Check sheet for the modelled part. Datum: model origin and axes. Units: mm. A direction names the side the tool comes from. Give positions to 0.01 mm unless a question says otherwise; leave off trailing zeros. Write each loop counter-clockwise with the first axis right and the second up, starting at its lowest first coordinate (ties: lowest second). Pieces come first, ordered by that corner, then holes. Notation, with made-up numbers: (72, 24) -> (76, 24) arc R21 cw to (76, 49) -> close; hole circle Ø7 at (21, 72.5). An arc over 180 degrees is marked (long way). Use a Markdown table: item, result. Add a question column.
1. Cross-section at D-D (x = 0). Enter the section's corners in (y, z), then the cut area to 3 significant figures.
2. Cross-section at B-B (x = 17.5). Enter the section's corners in (y, z), then the cut area to 3 significant figures.
3. Cross-section at A-A (y = -7). Enter the section's corners in (x, z), then the cut area to 3 significant figures.
4. Cross-section at C-C (z = 4.5). Count the separate pieces of the cut face and the enclosed holes in it, then the cut area to 3 significant figures.
5. Scan lines: probe 1 along X at (y, z) = (6, 4.5); probe 2 along Y at (x, z) = (0, 3.15); probe 3 along Y at (x, z) = (-30, 2.25). Record each from-to range of solid material in increasing order. Write a range as [from, to].
6. Set-up check for faces 1 (the cylindrical face through (-33.19, -23.09, 3.22)), 2 (the cylindrical face through (-0.86, 8.826, 3.846)), 3 (the flat face through (-11.15, 0, 3)): record each of +Z, -Z, +X, -X, +Y, -Y from which the full face is reachable in a straight line by a thin tool's end or side.
7. Release check for a two-part mould opening along X. For faces 4 (the cylindrical face through (-17.36, -19.05, 3.13)), 5 (the cylindrical face through (-33.19, 23.09, 3.22)), 6 (the cylindrical face through (33.09, -23.19, 3.22)) record: released by +X, released by -X, zero draft, split by the parting line, or undercut.
8. Gauge pin test, flat ends, axial feed: P1, Ø4, axis at x = 1, y = -11.5, coming from the +Z side; P2, Ø1, axis at x = 0, y = 11, coming from the -Z side. Record the tip position at first contact, or that the pin passes through.
from build123d import *

# Parameters (mm, degrees)
SKETCH1_W           = 70
SKETCH1_H           = 50
SKETCH1_R           = 1.397
SKETCH1_R_2         = 2.4892
BOSS_EXTRUDE1_DEPTH = 6.35
FILLET1_R           = 6.35
SKETCH3_R           = 3.96875
CUT_EXTRUDE1_DEPTH  = 5.08


with BuildPart() as part:
    # Sketch1 → Boss-Extrude1 (new body)
    with BuildSketch(Plane.XY):
        Rectangle(SKETCH1_W, SKETCH1_H)
        with Locations((30, 20)):
            Circle(SKETCH1_R, mode=Mode.SUBTRACT)
        with Locations((30, -20)):
            Circle(SKETCH1_R, mode=Mode.SUBTRACT)
        with Locations((-30, -20)):
            Circle(SKETCH1_R, mode=Mode.SUBTRACT)
        with Locations((-30, 20)):
            Circle(SKETCH1_R, mode=Mode.SUBTRACT)
        with Locations((0, 12.7)):
            Circle(SKETCH1_R_2, mode=Mode.SUBTRACT)
        with Locations((0, -12.7)):
            Circle(SKETCH1_R_2, mode=Mode.SUBTRACT)
        with BuildLine():
            Line((-23.85, -12.7), (-23.85, 12.7))
            ThreePointArc((-23.85, 12.7), (-17.5, 19.05), (-11.15, 12.7))
            Line((-11.15, 12.7), (-11.15, -12.7))
            ThreePointArc((-11.15, -12.7), (-17.5, -19.05), (-23.85, -12.7))
        make_face(mode=Mode.SUBTRACT)
        with BuildLine():
            Line((23.85, 12.7), (23.85, -12.7))
            ThreePointArc((23.85, -12.7), (17.5, -19.05), (11.15, -12.7))
            Line((11.15, -12.7), (11.15, 12.7))
            ThreePointArc((11.15, 12.7), (17.5, 19.05), (23.85, 12.7))
        make_face(mode=Mode.SUBTRACT)
    extrude(amount=BOSS_EXTRUDE1_DEPTH)

    # Fillet1
    fillet1_edges = [part.edges().sort_by_distance(p)[0] for p in [
        (-35, 25, 3.175),
        (35, 25, 3.175),
        (35, -25, 3.175),
        (-35, -25, 3.175),
    ]]
    fillet(fillet1_edges, radius=FILLET1_R)

    # Sketch3 → Cut-Extrude1 (cut)
    with BuildSketch(Plane.XY.offset(6.35)):
        with Locations((0, 12.7)):
            Circle(SKETCH3_R)
        with Locations((0, -12.7)):
            Circle(SKETCH3_R)
    extrude(amount=-CUT_EXTRUDE1_DEPTH, mode=Mode.SUBTRACT)


solid = part.part
Worked answers:
| question | item | result |
|---|---|---|
| 1 | outline | (-25, 0) -> (-15.19, 0) -> (-15.19, 1.27) -> (-16.67, 1.27) -> (-16.67, 6.35) -> (-25, 6.35) -> close; (-10.21, 0) -> (10.21, 0) -> (10.21, 1.27) -> (8.73, 1.27) -> (8.73, 6.35) -> (-8.73, 6.35) -> (-8.73, 1.27) -> (-10.21, 1.27) -> close; (15.19, 0) -> (25, 0) -> (25, 6.35) -> (16.67, 6.35) -> (16.67, 1.27) -> (15.19, 1.27) -> close |
| 1 | area | 224 mm² |
| 2 | outline | (-25, 0) -> (-19.05, 0) -> (-19.05, 6.35) -> (-25, 6.35) -> close; (19.05, 0) -> (25, 0) -> (25, 6.35) -> (19.05, 6.35) -> close |
| 2 | area | 75.6 mm² |
| 3 | outline | (-35, 0) -> (-23.85, 0) -> (-23.85, 6.35) -> (-35, 6.35) -> close; (-11.15, 0) -> (11.15, 0) -> (11.15, 6.35) -> (-11.15, 6.35) -> close; (23.85, 0) -> (35, 0) -> (35, 6.35) -> (23.85, 6.35) -> close |
| 3 | area | 283 mm² |
| 4 | separate pieces | 1 |
| 4 | enclosed holes | 8 |
| 4 | area | 2,440 mm² |
| 5 | probe 1 | x = [-35, -23.85], [-11.15, 11.15], [23.85, 35] |
| 5 | probe 2 | y = [-25, -16.67], [-8.73, 8.73], [16.67, 25] |
| 5 | probe 3 | y = [-24.85, -21.4], [-18.6, 18.6], [21.4, 24.85] |
| 6 | face 1 | +Z, -Z, -X, -Y |
| 6 | face 2 | +Z |
| 6 | face 3 | +Z, -Z |
| 7 | face 4 | undercut |
| 7 | face 5 | released by -X |
| 7 | face 6 | released by +X |
| 8 | P1 | stops at z = 1.27 |
| 8 | P2 | passes through |
